```python
from build123d import *
from build123d import SkipClean  # not in build123d's __all__

# Parameters (mm, degrees)
F0_R     = 2.5
F1_DEPTH = 152.4
F3_DEPTH = 16.5250114
F5_DEPTH = 16.5250114
F6_R     = 2.5
F7_DEPTH = 25.4
F9_DEPTH = 16.5250114


# Not quite as in the source:
# - after a boolean that leaves OpenCascade's solid faulty, fix() repairs it


with BuildPart() as f1:
    # F0 (on Top) → F1 (new body)
    with BuildSketch(Plane.XY):
        Circle(F0_R)
    extrude(amount=F1_DEPTH)

    # F2 (on face) → F3 (join)
    with BuildSketch(Plane.XY.offset(152.4)):
        with BuildLine():
            Line((0, -1.9312803396), (1.5875, -1.9312803396))
            ThreePointArc((1.5875, -1.9312803396), (0, 2.5), (-1.5875, -1.9312803396))
            Line((-1.5875, -1.9312803396), (0, -1.9312803396))
        make_face()
    extrude(amount=F3_DEPTH)

    # F4 (on face) → F5 (join)
    with BuildSketch(Plane(origin=(0, 0, 0), x_dir=(1, 0, 0), z_dir=(0, 0, -1))):
        with BuildLine():
            Line((1.5875, 1.9312803396), (-1.5875, 1.9312803396))
            ThreePointArc((-1.5875, 1.9312803396), (0, -2.5), (1.5875, 1.9312803396))
        make_face()
    with SkipClean():  # cleaning this boolean's faces spoils the solid; the shape is the same uncleaned
        extrude(amount=F5_DEPTH)

    # F6 (on face) → F7 (join)
    with BuildSketch(Plane(origin=(0, 0, -16.5250114), x_dir=(1, 0, 0), z_dir=(0, 0, -1))):
        Circle(F6_R)
    extrude(amount=F7_DEPTH)

    add(f1.part.fix(), mode=Mode.REPLACE)

    # F8 (on face) → F9 (join)
    with BuildSketch(Plane(origin=(0, 0, -41.9250114), x_dir=(1, 0, 0), z_dir=(0, 0, -1))):
        with BuildLine():
            Line((1.5875, 1.9312803396), (-1.5875, 1.9312803396))
            ThreePointArc((-1.5875, 1.9312803396), (0, -2.5), (1.5875, 1.9312803396))
        make_face()
    extrude(amount=F9_DEPTH)


solid = f1.part
```
Verification items for the finished model (mm, model axes). Coordinates: 2 decimals unless noted, no trailing zeros. Order: outer loops, then holes, each group sorted by start corner. A loop starts at its lowest first (then second) coordinate and runs counter-clockwise, first axis right, second up. Notation, with made-up numbers: (25, 3) -> (38, 3) arc R22 ccw to (38, 15) -> close; hole circle Ø10 at (46, 71). An arc over 180 degrees is marked (long way). Put each result on its own line as item: value. Start each with the question number.
1) Material ranges on L1, parallel to Z at x = 1.2, y = -2.1; L2, parallel to Y at x = -0.15, z = -37.5; L3, parallel to X at y = -0.45, z = 68.5, recorded low to high.
2) Cross-section at A-A (x = 0). Enter the section's corners in (y, z), plus the area to 3 significant figures.
3) Go/stop test with flat-tipped pins: pin 1 (1.5 mm diameter, centred on y = 1, z = 145, fed in from +X); pin 2 (1 mm diameter, centred on x = 0, z = -10, fed in from -Y); pin 3 (0.6 mm diameter, centred on x = -0.5, y = -2, fed in from -Z). Record where each tip stops, or that it passes through.
4) Cross-section at B-B (z = 130). Enter the section's corners in (x, y), plus the area to 3 significant figures.
Geometry check:
1. L1: z = -41.93 to -16.53, 0 to 152.4
1. L2: y = -2.5 to 2.5
1. L3: x = -2.46 to 2.46
2. outline: (-2.5, -41.93) -> (-1.93, -41.93) -> (-1.93, -58.45) -> (2.5, -58.45) -> (2.5, 168.93) -> (-1.93, 168.93) -> (-1.93, 152.4) -> (-2.5, 152.4) -> (-2.5, 0) -> (-1.93, 0) -> (-1.93, -16.53) -> (-2.5, -16.53) -> close
2. area: 1,110 mm^2
3. pin 1: stops at x = 2.49
3. pin 2: stops at y = -1.93
3. pin 3: stops at z = -58.45
4. outline: circle Ø5 at (0, 0)
4. area: 19.6 mm^2
